Input: part model. Units: mm. Frame: model coordinates. A direction names the side the tool comes from. Give positions to 0.01 mm unless a question says otherwise; leave off trailing zeros. Loops run counter-clockwise (first coordinate to the right, second up) from the corner with the lowest first, then second, coordinate; pieces in that order, holes last.
from build123d import *

# Parameters (mm, degrees)
F0_R     = 11
F1_DEPTH = 7
F3_DEPTH = 25
F4_R     = 5


with BuildPart() as f1:
    # F0 (on Top) → F1 (new body)
    with BuildSketch(Plane.XY):
        with BuildLine():
            Line((0, 19), (0, 14))
            ThreePointArc((0, 14), (-9.918883, 9.880068), (-13.999892, -0.054893))
            ThreePointArc((-13.999892, -0.054893), (-13.515832, -3.649971), (-12.124356, -7))
            ThreePointArc((-12.124356, -7), (-3.596948, -13.530039), (7.047485, -12.096816))
            ThreePointArc((7.047485, -12.096816), (9.918883, -9.880068), (12.124356, -7))
            ThreePointArc((12.124356, -7), (13.515832, 3.649971), (6.952408, 12.151709))
            Line((6.952408, 12.151709), (12.300835, 27.794118))
            ThreePointArc((12.300835, 27.794118), (-7.56054, 42.57536), (0, 19))
        make_face()
        Circle(F0_R, mode=Mode.SUBTRACT)
        with BuildLine():
            ThreePointArc((12.124356, -7), (9.918883, -9.880068), (7.047485, -12.096816))
            Line((7.047485, -12.096816), (17.919994, -24.549895))
            ThreePointArc((17.919994, -24.549895), (40.651613, -14.74006), (16.454483, -9.5))
            Line((16.454483, -9.5), (12.124356, -7))
        make_face()
        with BuildLine():
            ThreePointArc((-12.124356, -7), (-13.515832, -3.649971), (-13.999892, -0.054893))
            Line((-13.999892, -0.054893), (-30.22083, -3.244223))
            ThreePointArc((-30.22083, -3.244223), (-33.091073, -27.8353), (-16.454483, -9.5))
            Line((-16.454483, -9.5), (-12.124356, -7))
        make_face()
    extrude(amount=F1_DEPTH)

    # F2 (on face) → F3 (cut)
    with BuildSketch(Plane.XY.offset(7)):
        Polygon((5.435753, 41.415), (-5.435753, 41.415), (-10.871506, 32), (-5.435753, 22.585), (5.435753, 22.585), (10.871506, 32), align=None)
        Polygon((16.841307, -16), (22.27706, -25.415), (33.148566, -25.415), (38.584318, -16), (33.148566, -6.585), (22.27706, -6.585), align=None)
        Polygon((-22.27706, -6.585), (-33.148566, -6.585), (-38.584318, -16), (-33.148566, -25.415), (-22.27706, -25.415), (-16.841307, -16), align=None)
    extrude(amount=-F3_DEPTH, mode=Mode.SUBTRACT)

    # F4
    f4_edges = [f1.edges().sort_by_distance(p)[0] for p in [
        (6.952408, 12.151709, 3.5),
        (12.124356, -7, 3.5),
        (7.047485, -12.096816, 3.5),
        (-12.124356, -7, 3.5),
        (-13.999892, -0.054893, 3.5),
        (0, 14, 3.5),
    ]]
    fillet(f4_edges, radius=F4_R)


solid = f1.part
(1) Reachability of faces 1 (the flat face through (10.187, 21.612, 3.451)), 2 (the cylindrical face through (-10.052, 9.745, 3.451)), 3 (the cylindrical face through (13.742, -6.717, 3.549)) from +Z, -Z, +X, -X, +Y, -Y: full face, straight path, thin tool, end or side. Return the list, or none.
Values follow:
face 1: +Z, -Z, +X
face 2: +Z, -Z, -X
face 3: +Z, -Z
(2) Mould query, pull axis X, two halves, no side actions, for faces 4 (the flat face through (8.192, 36.642, 3.549)), 5 (the cylindrical face through (-1, 15.33, 3.55)), 6 (the flat face through (-3, 11, 0)). Classes: +X half, -X half, draft (parallel to the pull), parting line (faces both ways), or undercut.
Values follow:
face 4: undercut
face 5: -X half
face 6: draft
(3) Cut plane B-B (y = 40). Return the cut outline in (x, z).
Values follow:
outline: (-10.25, 0) - (-6.25, 0) - (-6.25, 7) - (-10.25, 7) - close; (6.25, 0) - (10.25, 0) - (10.25, 7) - (6.25, 7) - close
(4) Pin query (flat end, axial travel): pin 1 Ø3.5 at (x, z) = (29.5, 5) entering from +Y; pin 2 Ø4 at (y, z) = (24.5, 3.5) entering from +X; pin 3 Ø2 at (x, z) = (25.5, 3) entering from -Y. Return the tip coordinate at first contact, or that it passes through.
Values follow:
pin 1: stops at y = -3
pin 2: stops at x = 11.86
pin 3: stops at y = -28.94
(5) Cut plane C-C (z = 4). Count the separate pieces of the cut face and the enclosed holes in it, and give its area (3 significant figures).
Values follow:
separate pieces: 1
enclosed holes: 4
area: 1,110 mm2
(6) Cut plane A-A (x = -27.5). Return the cut outline in (y, z) (3 decimals).
Values follow:
outline: (-28.998, 0) - (-25.415, 0) - (-25.415, 7) - (-28.998, 7) - close; (-6.585, 0) - (-2.709, 0) - (-2.709, 7) - (-6.585, 7) - close
(7) Ray query, probe 1 along X at (y, z) = (-23, 6.5); probe 2 along Y at (x, z) = (-8.5, 6.5); probe 3 along X at (y, z) = (-20, 3.5). Return the intervals inside material, ascending.
Values follow:
probe 1: x = -38.67 to -34.54, -20.88 to -16.76, 16.57 to 20.88, 34.54 to 38.67
probe 2: y = -11.12 to -6.98, 6.98 to 11.12, 22.16 to 27.89, 36.11 to 41.84
probe 3: x = -40.08 to -36.27, -19.15 to -15.34, 13.95 to 19.15, 36.27 to 40.08
